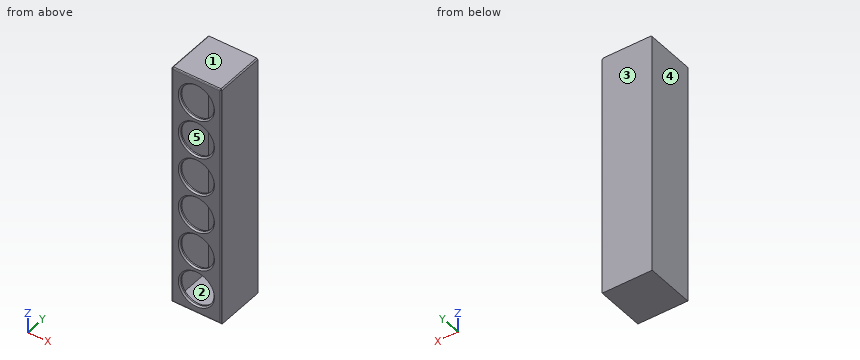
```python
from build123d import *

# Parameters (mm, degrees)
F0_W        = 228.6
F0_H        = 1117.6
F1_DEPTH    = 12.7
F3_DEPTH    = 203.2
F4_W        = 114.3
F4_H        = 1117.6
F5_DEPTH    = 12.7
F7_D        = 152.4
F7_DEPTH    = 25.4
F7_TIP      = 45.7855791699
F8_SIZE     = 5.08
F9_T1_DEPTH = 232.7728499247
F9_T3_DEPTH = 1121.7728499247


# Not quite as in the source:
# - a fillet or chamfer that OpenCascade refuses, or shapes differently, is made with other operations: its cross-section is extruded or revolved along the edge and cut away or added


with BuildPart() as f1:
    # F0 (on Front) → F1 (new body)
    with BuildSketch(Plane.XZ):
        Rectangle(F0_W, F0_H)
    extrude(amount=F1_DEPTH)

    # F2 (on face) → F3 (join)
    with BuildSketch(Plane.XZ.offset(12.7)):
        Polygon((-101.6, 546.1), (-114.3, 558.8), (-114.3, -558.8), (-101.6, -546.1), align=None)
        Polygon((114.3, 558.8), (-114.3, 558.8), (-101.6, 546.1), (101.6, 546.1), align=None)
        Polygon((114.3, -558.8), (114.3, 558.8), (101.6, 546.1), (101.6, -546.1), align=None)
        Polygon((-101.6, -546.1), (-114.3, -558.8), (114.3, -558.8), (101.6, -546.1), align=None)
    extrude(amount=F3_DEPTH)

    # F4 (on face) → F5 (join)
    with BuildSketch(Plane.XZ.offset(215.9)):
        with Locations((-57.15, 0)):
            Rectangle(F4_W, F4_H)
        with Locations((57.15, 0)):
            Rectangle(F4_W, F4_H)
    extrude(amount=F5_DEPTH)

    # F7
    with Locations(Plane.XZ.offset(228.6)):
        with Locations((0, -444.5), (0, -266.7), (0, -88.9), (0, 88.9), (0, 266.7), (0, 444.5)):
            Hole(F7_D / 2, depth=F7_DEPTH)
            with Locations((0, 0, -(F7_DEPTH + F7_TIP / 2))):  # 118° drill point
                Cone(0, F7_D / 2, F7_TIP, mode=Mode.SUBTRACT)

    # F8
    f8_edges = [f1.edges().sort_by_distance(p)[0] for p in [
        (0, -228.6, -558.8),
        (114.3, -228.6, 0),
        (-114.3, -228.6, 0),
        (0, -228.6, 558.8),
        (-114.3, -114.3, 558.8),
        (114.3, -114.3, 558.8),
    ]]
    chamfer(f8_edges, length=F8_SIZE)

    # F9: chamfer of 6.35 on 10 edges, made by hand

    # F9_s2 → F9_t1 (cut)
    with BuildSketch(Plane.YZ.offset(-116.3864249623)):
        Polygon((-226.7401280605, -555.5798719395), (-228.6, -551.0897438789), (-228.6, -553.72), align=None)
        Polygon((-228.6, 551.0897438789), (-226.7401280605, 555.5798719395), (-228.6, 553.72), align=None)
    extrude(amount=F9_T1_DEPTH, mode=Mode.SUBTRACT)

    # F9_s4 → F9_t3 (cut)
    with BuildSketch(Plane.XY.offset(-560.8864249623)):
        Polygon((-106.5897438789, -228.6), (-111.0798719395, -226.7401280605), (-109.22, -228.6), align=None)
        Polygon((111.0798719395, -226.7401280605), (106.5897438789, -228.6), (109.22, -228.6), align=None)
    extrude(amount=F9_T3_DEPTH, mode=Mode.SUBTRACT)

    # F9_s5 → F9_t6 (revolve, cut)
    with BuildSketch(Plane.XY.offset(-444.5)):
        Polygon((82.55, -228.6), (76.2, -222.25), (76.2, -228.6), align=None)
    revolve(axis=Axis((0, -228.6, -444.5), (0, -1, 0)), mode=Mode.SUBTRACT)

    # F9_s7 → F9_t8 (revolve, cut)
    with BuildSketch(Plane.XY.offset(-266.7)):
        Polygon((82.55, -228.6), (76.2, -222.25), (76.2, -228.6), align=None)
    revolve(axis=Axis((0, -228.6, -266.7), (0, -1, 0)), mode=Mode.SUBTRACT)

    # F9_s9 → F9_t10 (revolve, cut)
    with BuildSketch(Plane.XY.offset(-88.9)):
        Polygon((82.55, -228.6), (76.2, -222.25), (76.2, -228.6), align=None)
    revolve(axis=Axis((0, -228.6, -88.9), (0, -1, 0)), mode=Mode.SUBTRACT)

    # F9_s11 → F9_t12 (revolve, cut)
    with BuildSketch(Plane.XY.offset(88.9)):
        Polygon((82.55, -228.6), (76.2, -222.25), (76.2, -228.6), align=None)
    revolve(axis=Axis((0, -228.6, 88.9), (0, -1, 0)), mode=Mode.SUBTRACT)

    # F9_s13 → F9_t14 (revolve, cut)
    with BuildSketch(Plane.XY.offset(266.7)):
        Polygon((82.55, -228.6), (76.2, -222.25), (76.2, -228.6), align=None)
    revolve(axis=Axis((0, -228.6, 266.7), (0, -1, 0)), mode=Mode.SUBTRACT)

    # F9_s15 → F9_t16 (revolve, cut)
    with BuildSketch(Plane.XY.offset(444.5)):
        Polygon((82.55, -228.6), (76.2, -222.25), (76.2, -228.6), align=None)
    revolve(axis=Axis((0, -228.6, 444.5), (0, -1, 0)), mode=Mode.SUBTRACT)


solid = f1.part
```
The listing builds one solid part. Answer for the finished solid, in the listing's coordinates (mm). Face numbers are marked on the shaded views. A direction names the side the tool comes from. Coordinates: 2 decimals unless noted, no trailing zeros. Write each loop counter-clockwise with the first axis right and the second up, starting at its lowest first coordinate (ties: lowest second). Pieces come first, ordered by that corner, then holes. Notation, with made-up numbers: (24.5, -26) - (44.5, -26) arc R26 cw to (44.5, 11) - close; hole circle Ø3 at (57.5, 82). An arc over 180 degrees is marked (long way). Return JSON: item names as keys, results as strings. Group by question number.
1. Determine the mould class of the marked faces 1, 2 and 3 for opening direction Y: released by +Y, released by -Y, zero draft, split by the parting line, or undercut.
2. Straight lines are drawn through the part: L1, parallel to Z at x = -15, y = -65.5; L2, parallel to X at y = -219, z = 88; L3, parallel to X at y = -150.5, z = -210. For each, find the intervals that lie inside material, in ascending order.
3. A cutting plane is placed at C-C, the plane x = 0. Give the number of separate pieces and of enclosed holes in the cut face, plus the area to 3 significant figures.
4. Which of the six approach directions +Z, -Z, +X, -X, +Y, -Y give full straight-line access (tool end or side, diameter ignored) to the marked faces 4 and 5?
5. A cutting plane is placed at B-B, the plane z = 266.7. Determine the outline of the cut face in (x, y).
6. A cutting plane is placed at A-A, the plane y = -175.5. Determine the outline of the cut face in (x, z).
Ans:
{
 "1": {"face 1": "zero draft", "face 2": "undercut", "face 3": "released by +Y"},
 "2": {"L1": "-558.8 to -546.1, 546.1 to 558.8", "L2": "-114.3 to -76.19, 76.19 to 114.3", "L3": "-114.3 to -101.6, 101.6 to 114.3"},
 "3": {"separate pieces": "6", "enclosed holes": "0", "area": "21,700 mm²"},
 "4": {"face 4": "+Z, -Z, -X, +Y, -Y", "face 5": "none"},
 "5": {"outline": "(-114.3, -223.52) - (-111.08, -226.74) - (-106.59, -228.6) - (-82.55, -228.6) - (-76.2, -222.25) - (-76.2, -215.9) - (-101.6, -215.9) - (-101.6, -12.7) - (101.6, -12.7) - (101.6, -215.9) - (76.2, -215.9) - (76.2, -222.25) - (82.55, -228.6) - (106.59, -228.6) - (111.08, -226.74) - (114.3, -223.52) - (114.3, 0) - (-114.3, 0) - close"},
 "6": {"outline": "(-114.3, -558.8) - (114.3, -558.8) - (114.3, 553.72) - (109.22, 558.8) - (-109.22, 558.8) - (-114.3, 553.72) - close; hole (-101.6, -546.1) - (101.6, -546.1) - (101.6, 546.1) - (-101.6, 546.1) - close"}
}
